Could you check a few things on this model? Use its own coordinates, in mm. A direction names the side the tool comes from. Give positions to 0.01 mm unless a question says otherwise; leave off trailing zeros. Use CSV: the item, a comma, the result in double quotes.
```python
from build123d import *

# Parameters (mm, degrees)
SWEEP1_PROFILE_R     = 6.35
CUT_SWEEP1_PROFILE_R = 3.175


with BuildPart() as part:
    # Sweep1: sweep along a curve in space
    with BuildLine() as sweep1_path:
        Line((-25.144717139, 46.783, -16.764999998), (-25.144717139, 46.783, 0))
        ThreePointArc((-25.144717139, 46.783, 0), (-37.539812947, 54.270144781, 98.408776247), (-73.67428039, 76.09684088, 188.474744178))
        ThreePointArc((-77.762208871, 65.122942343, 288.925037219), (-87.944554744, 81.01650581, 239.339220312), (-73.67428039, 76.09684088, 188.474744178))
        Line((-68.87554044, 55.005914395, 306.16579471), (-77.762208871, 65.122942343, 288.925037219))
    # Sweep1 profile (on start of the path) → Sweep1 (sweep)
    with BuildSketch(Plane(origin=(-25.144717139, 46.783, -16.764999998), x_dir=(1, 0, 0), z_dir=(0, 0, 1))):
        Circle(SWEEP1_PROFILE_R)
    sweep(path=sweep1_path.line)

    # Cut-Sweep1: sweep along a curve in space
    with BuildLine() as cut_sweep1_path:
        Line((-25.144717139, 46.783, -16.764999998), (-25.144717139, 46.783, 0))
        ThreePointArc((-25.144717139, 46.783, 0), (-37.539812947, 54.270144781, 98.408776247), (-73.67428039, 76.09684088, 188.474744178))
        ThreePointArc((-77.762208871, 65.122942343, 288.925037219), (-87.944554744, 81.01650581, 239.339220312), (-73.67428039, 76.09684088, 188.474744178))
        Line((-68.87554044, 55.005914395, 306.16579471), (-77.762208871, 65.122942343, 288.925037219))
    # Cut-Sweep1 profile (on start of the path) → Cut-Sweep1 (sweep, cut)
    with BuildSketch(Plane(origin=(-25.144717139, 46.783, -16.764999998), x_dir=(1, 0, 0), z_dir=(0, 0, 1))):
        Circle(CUT_SWEEP1_PROFILE_R)
    sweep(path=cut_sweep1_path.line, mode=Mode.SUBTRACT)


solid = part.part
```
1. If we mould it in two halves opening along Y, with no side actions, what happens to faces 1 (the face through (-75.303, 61.475, 299.59)), 2 (the face through (-66.378, 57.925, 306.592)), 3 (the face through (-28, 45, -16.765)), 4 (the face through (-27.7, 44.9, -8.3))? For each: +Y half, -Y half, draft (parallel to the pull), parting line (faces both ways), or undercut.
Outcome:
face 1,"undercut"
face 2,"-Y half"
face 3,"draft"
face 4,"undercut"
2. Please list where these lines run through material, in increasing order: line 1 (Z direction, x = -65.5, y = 69.5); line 2 (Z direction, x = -75, y = 75); line 3 (X direction, y = 83, z = 220.5).
Outcome:
line 1,"159.04 to 165.99, 177.29 to 183.71"
line 2,"178.01 to 184.36, 194.63 to 202.01"
line 3,"-91.97 to -88.59, -82.65 to -79.26"
3. I'm going to push flat-ended pins straight in: pin 1 Ø1.5 at (x, y) = (-82, 73) entering from +Z; pin 2 Ø5 at (y, z) = (56, 126.5) entering from -X; pin 3 Ø4 at (y, z) = (78.5, 171.5) entering from -X. Where does each tip first touch, or does it pass through?
Outcome:
pin 1,"z = 288.35"
pin 2,"x = -52.82"
pin 3,"x = -69.4"
4. Which directions (+Z, -Z, +X, -X, +Y, -Y) give clear straight access to the entire face, cutting with the end or side of a thin tool? Please do faces 5 (the face through (-77.35, 62.96, 301.51)), 6 (the face through (-26.521, 40.584, -8.265)).
Outcome:
face 5,"none"
face 6,"-Z"
